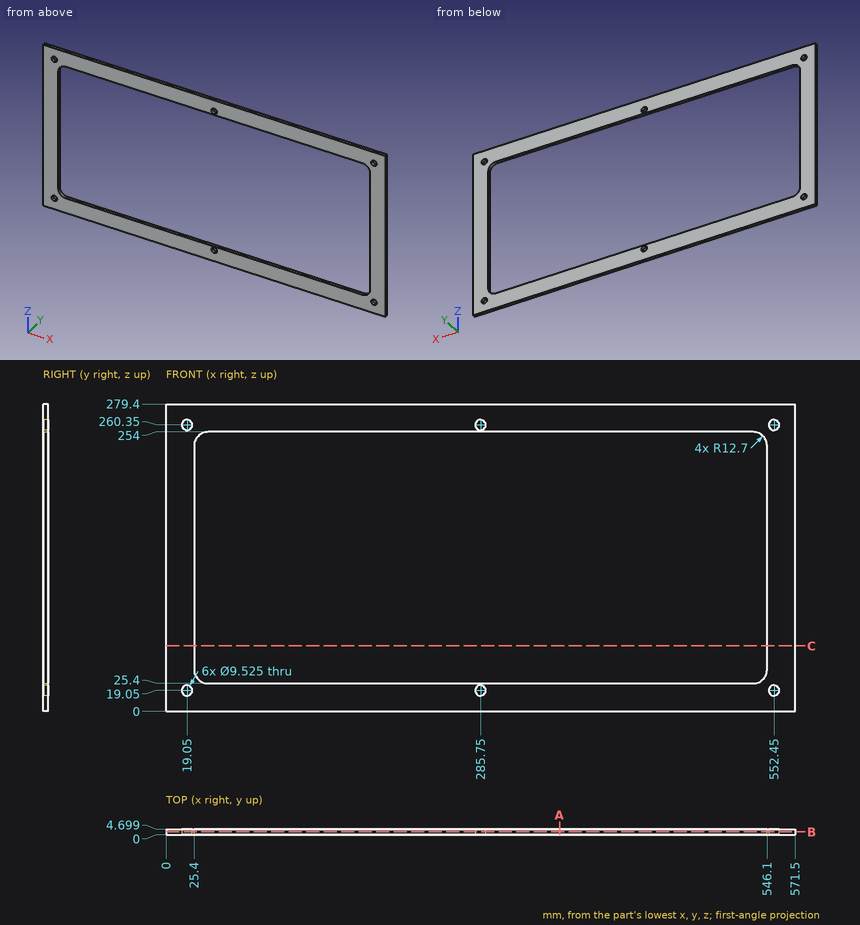
For this review, use the dimensioned drawing (mm, ordinates from the lowest corner) and the shaded views. Give positions to 0.01 mm unless a question says otherwise; leave off trailing zeros. Write each loop counter-clockwise with the first axis right and the second up, starting at its lowest first coordinate (ties: lowest second). Pieces come first, ordered by that corner, then holes. Notation, with made-up numbers: M 57,-22.75 L 98,-22.75 A35 ccw 98,9.25 Z; hole C 24,-40 d11. An arc over 180 degrees is marked long. Answer as a JSON object with one key per item and string values. Group by question number.
Item 1: Consider section C-C on z = 59.5. Write out the cut boundary in (x, y).
Item 2: Consider section A-A on x = 357.5. Write out the cut boundary in (y, z).
Item 3: For probe 1 along Z at (x, y) = (552.45, 2.65); probe 2 along X at (y, z) = (2.65, 260.35); probe 3 along Z at (x, y) = (285.75, 2.1), list the stretches that pass through material, from the lowest coordinate up. Write a range as [from, to].
Item 4: For pin 1 Ø7.5 at (x, z) = (285.75, 260.35) entering from +Y; pin 2 Ø15 at (x, z) = (285.75, 19.05) entering from -Y, all flat-tipped, find the tip position at first contact; note any pin that passes through.
Item 5: Consider section B-B on y = 2.4. Count the separate pieces of the cut face and the enclosed holes in it, plus the area to 3 significant figures.
Check result:
{
 "1": {"outline": "M 0,0 L 25.4,0 L 25.4,4.7 L 0,4.7 Z; M 546.1,0 L 571.5,0 L 571.5,4.7 L 546.1,4.7 Z"},
 "2": {"outline": "M 0,0 L 4.7,0 L 4.7,25.4 L 0,25.4 Z; M 0,254 L 4.7,254 L 4.7,279.4 L 0,279.4 Z"},
 "3": {"probe 1": "z = [0, 14.29], [23.81, 255.59], [265.11, 279.4]", "probe 2": "x = [0, 14.29], [23.81, 280.99], [290.51, 547.69], [557.21, 571.5]", "probe 3": "z = [0, 14.29], [23.81, 25.4], [254, 255.59], [265.11, 279.4]"},
 "4": {"pin 1": "passes through", "pin 2": "stops at y = 0"},
 "5": {"separate pieces": "1", "enclosed holes": "7", "area": "40,400 mm^2"}
}
